For this review, take the finished solid that the model builds, in its own axes (mm). A direction names the side the tool comes from. Coordinates: 2 decimals unless noted, no trailing zeros. Write each loop counter-clockwise with the first axis right and the second up, starting at its lowest first coordinate (ties: lowest second). Pieces come first, ordered by that corner, then holes. Notation, with made-up numbers: (33.5, 20.5) -> (79.5, 20.5) arc R29 cw to (79.5, 42.5) -> close; hole circle Ø10 at (53.25, 12). An arc over 180 degrees is marked (long way). One line per item, written item: value. Start each with the question number.
1) For probe 1 along Y at (x, z) = (-47, -5); probe 2 along X at (y, z) = (-11, -11.25); probe 3 along Y at (x, z) = (-36, -11.5), list the stretches that pass through material, from the lowest coordinate up. Write a range as from..to.
2) Add section A-A (x = 41). State the section outline as (y, z) points.
3) Add section D-D (y = -14.5). State the section outline as (x, z) points, and give its area (3 significant figures).
4) For pin 1 Ø6 at (x, z) = (-34.5, -11.5) entering from +Y; pin 2 Ø3 at (y, z) = (1.5, -12) entering from -X; pin 3 Ø4 at (y, z) = (-4, -8) entering from +X, all flat-tipped, find the tip position at first contact; note any pin that passes through.
5) Machinability: for faces 1 (the flat face through (-45, -9.3, -11.7)), 2 (the flat face through (-47, -9, -12)), 3 (the flat face through (-10, 14, -3)), 4 (the flat face through (30, -15, -24)), which of the approach directions +Z, -Z, +X, -X, +Y, -Y give a long, thin tool a straight path to every point of the face, cutting with its end or side? Answer none if there is none.
6) Mouldability with a two-part tool opening along X and no side actions: class faces 5 (the flat face through (-49, -9.3, -11.7)), 6 (the flat face through (30, -15, -2)), 7 (the flat face through (-30, -15, -24)), 8 (the flat face through (-8, 13, 0)) as released by +X, released by -X, zero draft, split by the parting line, or undercut.
7) Add section C-C (x = -47). State the section outline as (y, z) points.
8) Add section B-B (y = 11). State the section outline as (x, z) points, and give its area (3 significant figures).
from build123d import *

# Parameters (mm, degrees)
SKETCH_1_W          = 98
SKETCH_1_H          = 33
SKETCH_1_W_2        = 90
SKETCH_1_H_2        = 25
EXTRUDE_1_DEPTH     = 25.05
SKETCH_2_W          = 5.5
SKETCH_2_H          = 5.5
EXTRUDE_2_DEPTH     = 25.05
SKETCH_3_W          = 5.5
SKETCH_3_H          = 5.5
EXTRUDE_3_DEPTH     = 25.05
SKETCH_4_W          = 5.5
SKETCH_4_H          = 5.5
EXTRUDE_4_DEPTH     = 25.05
SKETCH_5_W          = 5.5
SKETCH_5_H          = 5.5
EXTRUDE_5_DEPTH     = 25.05
SKETCH_6_R          = 1.6
CUT_EXTRUDE_1_DEPTH = 25.05
SKETCH_7_W          = 4
SKETCH_7_H          = 19.05
CUT_EXTRUDE_2_DEPTH = 4
SKETCH_8_W          = 4
SKETCH_8_H          = 19.05
SKETCH_8_H_2        = 13.5
CUT_EXTRUDE_3_DEPTH = 4
SKETCH_9_W          = 23.05
SKETCH_9_H          = 18
CUT_EXTRUDE_4_DEPTH = 4
SKETCH_10_W         = 60
SKETCH_10_H         = 4.5
CUT_EXTRUDE_5_DEPTH = 25.05
CUT_EXTRUDE_6_DEPTH = 4


with BuildPart() as part:
    # 草图1 → 凸台-拉伸1 (new body)
    with BuildSketch(Plane.XY.offset(-25.05)):
        Rectangle(SKETCH_1_W, SKETCH_1_H)
        Rectangle(SKETCH_1_W_2, SKETCH_1_H_2, mode=Mode.SUBTRACT)
    extrude(amount=EXTRUDE_1_DEPTH)

    # 草图2 → 凸台-拉伸2 (add)
    with BuildSketch(Plane.XY.offset(-25.05)):
        with Locations((47.75, 15.25)):
            Rectangle(SKETCH_2_W, SKETCH_2_H)
    extrude(amount=EXTRUDE_2_DEPTH)

    # 草图3 → 凸台-拉伸3 (add)
    with BuildSketch(Plane.XY.offset(-25.05)):
        with Locations((47.75, -15.25)):
            Rectangle(SKETCH_3_W, SKETCH_3_H)
    extrude(amount=EXTRUDE_3_DEPTH)

    # 草图4 → 凸台-拉伸4 (add)
    with BuildSketch(Plane.XY.offset(-25.05)):
        with Locations((-47.75, 15.25)):
            Rectangle(SKETCH_4_W, SKETCH_4_H)
    extrude(amount=EXTRUDE_4_DEPTH)

    # 草图5 → 凸台-拉伸5 (add)
    with BuildSketch(Plane.XY.offset(-25.05)):
        with Locations((-47.75, -15.25)):
            Rectangle(SKETCH_5_W, SKETCH_5_H)
    extrude(amount=EXTRUDE_5_DEPTH)

    # 草图6 → 切除-拉伸1 (cut)
    with BuildSketch(Plane.XY.offset(-25.05)):
        with Locations((-47, -14.5)):
            Circle(SKETCH_6_R)
        with Locations((-47, 14.5)):
            Circle(SKETCH_6_R)
        with Locations((47, -14.5)):
            Circle(SKETCH_6_R)
        with Locations((47, 14.5)):
            Circle(SKETCH_6_R)
    extrude(amount=CUT_EXTRUDE_1_DEPTH, mode=Mode.SUBTRACT)

    # 草图7 → 切除-拉伸2 (cut)
    with BuildSketch(Plane(origin=(0, -16.5, 0), x_dir=(1, 0, 0), z_dir=(0, 1, 0))):
        with Locations((-30, 12.525)):
            Rectangle(SKETCH_7_W, SKETCH_7_H)
        with Locations((-20, 12.525)):
            Rectangle(SKETCH_7_W, SKETCH_7_H)
        with Locations((-10, 12.525)):
            Rectangle(SKETCH_7_W, SKETCH_7_H)
        with Locations((0, 12.525)):
            Rectangle(SKETCH_7_W, SKETCH_7_H)
        with Locations((10, 12.525)):
            Rectangle(SKETCH_7_W, SKETCH_7_H)
        with Locations((20, 12.525)):
            Rectangle(SKETCH_7_W, SKETCH_7_H)
        with Locations((30, 12.525)):
            Rectangle(SKETCH_7_W, SKETCH_7_H)
    extrude(amount=CUT_EXTRUDE_2_DEPTH, mode=Mode.SUBTRACT)

    # 草图8 → 切除-拉伸3 (cut)
    with BuildSketch(Plane(origin=(0, 12.5, 0), x_dir=(1, 0, 0), z_dir=(0, 1, 0))):
        with Locations((-30, 12.525)):
            Rectangle(SKETCH_8_W, SKETCH_8_H)
        with Locations((-20, 12.525)):
            Rectangle(SKETCH_8_W, SKETCH_8_H)
        with Locations((-10, 9.75)):
            Rectangle(SKETCH_8_W, SKETCH_8_H_2)
        with Locations((0, 9.75)):
            Rectangle(SKETCH_8_W, SKETCH_8_H_2)
        with Locations((10, 9.75)):
            Rectangle(SKETCH_8_W, SKETCH_8_H_2)
        with Locations((20, 12.525)):
            Rectangle(SKETCH_8_W, SKETCH_8_H)
        with Locations((30, 12.525)):
            Rectangle(SKETCH_8_W, SKETCH_8_H)
    extrude(amount=CUT_EXTRUDE_3_DEPTH, mode=Mode.SUBTRACT)

    # 草图9 → 切除-拉伸4 (cut)
    with BuildSketch(Plane(origin=(-49, 0, 0), x_dir=(0, 0, -1), z_dir=(1, 0, 0))):
        with Locations((12.525, 0)):
            Rectangle(SKETCH_9_W, SKETCH_9_H)
    extrude(amount=CUT_EXTRUDE_4_DEPTH, mode=Mode.SUBTRACT)

    # 草图10 → 切除-拉伸5 (cut)
    with BuildSketch(Plane.XY.offset(-25.05)):
        with Locations((0, -14.75)):
            Rectangle(SKETCH_10_W, SKETCH_10_H)
    extrude(amount=CUT_EXTRUDE_5_DEPTH, mode=Mode.SUBTRACT)

    # 草图11 → 切除-拉伸6 (cut)
    with BuildSketch(Plane(origin=(0, 12.5, 0), x_dir=(1, 0, 0), z_dir=(0, 1, 0))):
        with BuildLine():
            Line((-8, 17.82), (8, 17.82))
            ThreePointArc((8, 17.82), (11, 20.82), (8, 23.82))
            Line((8, 23.82), (-8, 23.82))
            ThreePointArc((-8, 23.82), (-11, 20.82), (-8, 17.82))
        make_face()
    extrude(amount=CUT_EXTRUDE_6_DEPTH, mode=Mode.SUBTRACT)


solid = part.part
Numbers:
1. probe 1: -18..-16.1, -12.9..-9, 9..12.9, 16.1..18
1. probe 2: -49..-45, 45..49
1. probe 3: -16.5..-12.5, 12.5..16.5
2. outline: (-16.5, -25.05) -> (-12.5, -25.05) -> (-12.5, 0) -> (-16.5, 0) -> close; (12.5, -25.05) -> (16.5, -25.05) -> (16.5, 0) -> (12.5, 0) -> close
3. outline: (-50.5, -25.05) -> (-48.6, -25.05) -> (-48.6, 0) -> (-50.5, 0) -> close; (-45.4, -25.05) -> (-30, -25.05) -> (-30, -22.05) -> (-32, -22.05) -> (-32, -3) -> (-30, -3) -> (-30, 0) -> (-45.4, 0) -> close; (30, -25.05) -> (45.4, -25.05) -> (45.4, 0) -> (30, 0) -> (30, -3) -> (32, -3) -> (32, -22.05) -> (30, -22.05) -> close; (48.6, -25.05) -> (50.5, -25.05) -> (50.5, 0) -> (48.6, 0) -> close
3. area: 791 mm²
4. pin 1: y = 16.5
4. pin 2: x = 45
4. pin 3: x = 49
5. face 1: +Z, -Z
5. face 2: -X
5. face 3: +Y, -Y
5. face 4: +Z, -Z, -Y
6. face 5: released by -X
6. face 6: undercut
6. face 7: undercut
6. face 8: zero draft
7. outline: (-18, -25.05) -> (-16.1, -25.05) -> (-16.1, 0) -> (-18, 0) -> close; (-12.9, -25.05) -> (12.9, -25.05) -> (12.9, 0) -> (-12.9, 0) -> close; (16.1, -25.05) -> (18, -25.05) -> (18, 0) -> (16.1, 0) -> close; hole (-9, -24.05) -> (9, -24.05) -> (9, -1) -> (-9, -1) -> close
8. outline: (-49, -25.05) -> (-45, -25.05) -> (-45, 0) -> (-49, 0) -> close; (45, -25.05) -> (49, -25.05) -> (49, 0) -> (45, 0) -> close
8. area: 200 mm²
